```python
from build123d import *

# Parameters (mm, degrees)
SKETCH1_W                                      = 9.525
SKETCH1_H                                      = 25.4
BOSS_EXTRUDE1_DEPTH                            = 450.85
CBORE_FOR_8_SOCKET_HEAD_CAP_SCREW1_D           = 4.9149
CBORE_FOR_8_SOCKET_HEAD_CAP_SCREW1_CBORE_D     = 7.9375
CBORE_FOR_8_SOCKET_HEAD_CAP_SCREW1_CBORE_DEPTH = 5.4356
CBORE_FOR_8_SOCKET_HEAD_CAP_SCREW2_D           = 4.9149
CBORE_FOR_8_SOCKET_HEAD_CAP_SCREW2_CBORE_D     = 7.9375
CBORE_FOR_8_SOCKET_HEAD_CAP_SCREW2_CBORE_DEPTH = 16.8656
F_8_32_TAPPED_HOLE1_D                          = 3.4544


with BuildPart() as part:
    # Sketch1 → Boss-Extrude1 (new body)
    with BuildSketch(Plane(origin=(0, 0, 0), x_dir=(1, 0, 0), z_dir=(0, 1, 0))):
        with Locations((-8.211890298, -2.158307883)):
            Rectangle(SKETCH1_W, SKETCH1_H)
    extrude(amount=BOSS_EXTRUDE1_DEPTH)

    # CBORE for #8 Socket Head Cap Screw1 (through all)
    with Locations(Plane.ZY.offset(12.974390298)):
        with Locations((10.095807883, 41.275), (10.095807883, 114.935), (10.095807883, 188.595), (10.095807883, 262.255), (10.095807883, 335.915), (10.095807883, 409.575)):
            CounterBoreHole(CBORE_FOR_8_SOCKET_HEAD_CAP_SCREW1_D / 2, CBORE_FOR_8_SOCKET_HEAD_CAP_SCREW1_CBORE_D / 2, CBORE_FOR_8_SOCKET_HEAD_CAP_SCREW1_CBORE_DEPTH)

    # CBORE for #8 Socket Head Cap Screw2 (through all)
    with Locations(Plane(origin=(0, 0, -10.541692117), x_dir=(-1, 0, 0), z_dir=(0, 0, -1))):
        with Locations((8.211890298, 6.35), (8.211890298, 19.05), (8.211890298, 431.8), (8.211890298, 444.5)):
            CounterBoreHole(CBORE_FOR_8_SOCKET_HEAD_CAP_SCREW2_D / 2, CBORE_FOR_8_SOCKET_HEAD_CAP_SCREW2_CBORE_D / 2, CBORE_FOR_8_SOCKET_HEAD_CAP_SCREW2_CBORE_DEPTH)

    # #8-32 Tapped Hole1 (through all)
    with Locations(Plane.ZY.offset(12.974390298)):
        with Locations((-4.191692117, 41.275), (-4.191692117, 114.935), (-4.191692117, 188.595), (-4.191692117, 262.255), (-4.191692117, 335.915), (-4.191692117, 409.575)):
            Hole(F_8_32_TAPPED_HOLE1_D / 2)


solid = part.part
```
Geometry: final body of the model. Coordinates: model frame, mm. A direction names the side the tool comes from. Coordinates: 2 decimals unless noted, no trailing zeros. Order: outer loops, then holes, each group sorted by start corner. A loop starts at its lowest first (then second) coordinate and runs counter-clockwise, first axis right, second up. Notation, with made-up numbers: (-4, 80) -> (14, 80) arc R21 cw to (14, 112) -> close; hole circle Ø10 at (10, 57.25). An arc over 180 degrees is marked (long way). Use CSV: the item, a comma, the result in double quotes.
1) Access query for faces 4 (the cylindrical face through (-10.29, 405.7, 9.24)), 5 (the flat face through (-11, 6, 6.324)), 6 (the flat face through (-8, 0, 2)). Directions: +Z, -Z, +X, -X, +Y, -Y. A direction counts if a zero-diameter tool reaches every point of the face in a straight line with its end or side. Return the directions, or none.
Findings:
face 4,"-X"
face 5,"-Z"
face 6,"+Z, -Z, +X, -X, -Y"
2) Section A-A on z = 2.25. Output: boundary loops of the cut face in (x, y).
Findings:
outline,"(-12.97, 0) -> (-3.45, 0) -> (-3.45, 450.85) -> (-12.97, 450.85) -> close; hole circle Ø7.94 at (-8.21, 6.35); hole circle Ø7.94 at (-8.21, 19.05); hole circle Ø7.94 at (-8.21, 431.8); hole circle Ø7.94 at (-8.21, 444.5)"
3) Mould query, pull axis Y, two halves, no side actions, for faces 1 (the flat face through (-12.974, 222, 2)), 2 (the cylindrical face through (-10.29, 258.38, 9.24)), 3 (the flat face through (-8, 450.85, 2)). Classes: +Y half, -Y half, draft (parallel to the pull), parting line (faces both ways), or undercut.
Findings:
face 1,"draft"
face 2,"undercut"
face 3,"+Y half"
4) Line query: line 1 (Y direction, x = -5.5, z = 3); line 2 (Y direction, x = -11.5, z = 2.75); line 3 (Z direction, x = -9.25, y = 42). Output: solid intervals per line, ascending.
Findings:
line 1,"y = 0 to 3.45, 9.25 to 16.15, 21.95 to 428.9, 434.7 to 441.6, 447.4 to 450.85"
line 2,"y = 0 to 4.13, 8.57 to 16.83, 21.27 to 429.58, 434.02 to 442.28, 446.72 to 450.85"
line 3,"z = -10.54 to -5.76, -2.62 to 6.19, 14 to 14.86"
5) Pin query (flat end, axial travel): pin 1 Ø4 at (x, y) = (-8.21, 431.8) entering from +Z; pin 2 Ø4 at (y, z) = (261.5, 8.5) entering from -X. Return the tip coordinate at first contact, or that it passes through.
Findings:
pin 1,"passes through"
pin 2,"stops at x = -7.54"
